Can you work these out from the model? Positions are in its coordinate system, mm. A direction names the side the tool comes from. Give positions to 0.01 mm unless a question says otherwise; leave off trailing zeros. Order: outer loops, then holes, each group sorted by start corner. A loop starts at its lowest first (then second) coordinate and runs counter-clockwise, first axis right, second up. Notation, with made-up numbers: M 5,58 L 13,58 A12 ccw 13,62 Z; hole C 64.5,42 d4. An arc over 180 degrees is marked long. Use a Markdown table: item, result. Add a question column.
from build123d import *

# Parameters (mm, degrees)
EXTRUDE1_DEPTH              = 12.7
ARC_MOUNTING_SLOT_I_DEPTH   = 56.885195213
CLAMPING_SCREW_HOLES_D      = 5.1054
CLAMPING_SCREW_HOLES_DEPTH  = 21.59
CLAMPING_SCREW_HOLES_TIP    = 1.533816902
SKETCH7_R                   = 9.525
CUT_EXTRUDE1_DEPTH          = 38.862
CUT_EXTRUDE2_DEPTH          = 25.4
ADVANCEDHOLE1_START         = -12.7
ADVANCEDHOLE1_OUTLINE_R     = 2.5527
ADVANCEDHOLE1_DEPTH         = 25.4
ADVANCEDHOLE1_2_OUTLINE_R   = 3.2639
ADVANCEDHOLE1_2_OUTLINE_R_2 = 2.5527
ADVANCEDHOLE1_2_DEPTH       = 11.1125
FILLET1_R                   = 1.5875


# Read off the part's stored shape, not the designer's step: AdvancedHole1
with BuildPart() as part:
    # Sketch1 → Extrude1 (new, symmetric)
    with BuildSketch(Plane.XY):
        Polygon((-28.575, 0), (-28.575, 6.35), (-38.1, 6.35), (-38.1, 16.1036), (-38.1, 54.9656), (-12.7, 54.9656), (10.16, 54.9656), (10.16, 33.3756), (0, 33.3756), (0, 16.1036), (12.7, 16.1036), (31.75, 16.1036), (31.75, 0), align=None)
    extrude(amount=EXTRUDE1_DEPTH, both=True)

    # Sketch2 → Arc mounting slot I (cut, through all)
    with BuildSketch(Plane(origin=(0, 16.1036, 0), x_dir=(-1, 0, 0), z_dir=(0, 1, 0))):
        with BuildLine():
            ThreePointArc((-25.839582785, -4.556215615), (-21.92608696, -7.296474893), (-19.185827683, -3.382979068))
            ThreePointArc((-19.185827683, -3.382979068), (-19.4818, 0), (-19.185827683, 3.382979068))
            ThreePointArc((-19.185827683, 3.382979068), (-21.92608696, 7.296474893), (-25.839582785, 4.556215615))
            ThreePointArc((-25.839582785, 4.556215615), (-26.2382, 0), (-25.839582785, -4.556215615))
        make_face()
    arc_mounting_slot_i = extrude(amount=-ARC_MOUNTING_SLOT_I_DEPTH, mode=Mode.SUBTRACT)

    # Arc mounting slot II: Arc mounting slot I across plane
    add(arc_mounting_slot_i.mirror(Plane(origin=(0, 0, 0), x_dir=(0, 0, 1), z_dir=(1, 0, 0))), mode=Mode.SUBTRACT)

    # Clamping screw holes
    with Locations(Plane(origin=(0, 54.9656, 0), x_dir=(-1, 0, 0), z_dir=(0, 1, 0))):
        with Locations((-3.96875, -7.9375), (-3.96875, 7.9375)):
            Hole(CLAMPING_SCREW_HOLES_D / 2, depth=CLAMPING_SCREW_HOLES_DEPTH)
            with Locations((0, 0, -(CLAMPING_SCREW_HOLES_DEPTH + CLAMPING_SCREW_HOLES_TIP / 2))):  # 118° drill point
                Cone(0, CLAMPING_SCREW_HOLES_D / 2, CLAMPING_SCREW_HOLES_TIP, mode=Mode.SUBTRACT)

    # Sketch7 → Cut-Extrude1 (cut)
    with BuildSketch(Plane(origin=(0, 54.9656, 0), x_dir=(1, 0, 0), z_dir=(0, 1, 0))):
        with Locations(Location((-19.05, 0, 0), (0, 0, 270))):
            Circle(SKETCH7_R)
    extrude(amount=-CUT_EXTRUDE1_DEPTH, mode=Mode.SUBTRACT)

    # Sketch9 → Cut-Extrude2 (cut)
    with BuildSketch(Plane.ZY.offset(38.1)):
        Polygon((-1.5875, 19.2786), (-1.5875, 54.9656), (1.5875, 54.9656), (1.5875, 16.1036), (-12.7, 16.1036), (-12.7, 19.2786), align=None)
    extrude(amount=-CUT_EXTRUDE2_DEPTH, mode=Mode.SUBTRACT)

    # AdvancedHole1 outline → AdvancedHole1 (cut)
    with BuildSketch(Plane.XY.offset(ADVANCEDHOLE1_START)):
        with Locations((-33.270888328, 37.1221)):
            Circle(ADVANCEDHOLE1_OUTLINE_R)
    extrude(amount=ADVANCEDHOLE1_DEPTH, mode=Mode.SUBTRACT)

    # AdvancedHole1 2 outline → AdvancedHole1 2 (cut)
    with BuildSketch(Plane.XY.offset(ADVANCEDHOLE1_START)):
        with Locations((-33.270888328, 37.1221)):
            Circle(ADVANCEDHOLE1_2_OUTLINE_R)
        with Locations((-33.270888328, 37.1221)):
            Circle(ADVANCEDHOLE1_2_OUTLINE_R_2, mode=Mode.SUBTRACT)
    extrude(amount=ADVANCEDHOLE1_2_DEPTH, mode=Mode.SUBTRACT)

    # Fillet1
    fillet1_edges = [part.edges().sort_by_distance(p)[0] for p in [
        (-12.7, 19.2786, -9.899757914),
        (-12.7, 16.1036, -9.899757914),
        (-33.270888328, 16.1036, 1.5875),
    ]]
    fillet(fillet1_edges, radius=FILLET1_R - 0.0001)  # a hair under: the kernel refuses the full size


solid = part.part
1. If we section it at D-D, the plane y = 14.5: List the corners of the cut face in (x, z) for me, then the cut area to 3 significant figures.
2. We'd pull the mould along Z, two halves only. Please class faces 6 (the face through (-19.48, 8.16, -0.05)), 7 (the face through (-10, 28, -12.7)), 8 (the face through (10.16, 44, 0)): +Z half, -Z half, draft (parallel to the pull), parting line (faces both ways), or undercut.
3. If we section it at B-B, the plane x = -23: List the corners of the cut face in (y, z) for me.
4. If we section it at A-A, the plane y = 5: List the corners of the cut face in (x, z) for me (3 decimals).
5. I need wall thicknesses on L1, parallel to X at y = 38.5, z = -4.5; L2, parallel to X at y = 38.5, z = -2; L3, parallel to Y at x = -33.5, z = 7. Which ranges of each line are inside material? Lowest first, please. Write a range as [from, to].
6. Will this pin go through, and if not, where does the flat tip stop? pin 1 (5 mm diameter, centred on x = -33, z = -5, fed in from -Y).
7. If we section it at C-C, the plane x = -16: List the corners of the cut face in (y, z) for me, then the cut area to 3 significant figures.
8. On a 3-axis mill with a long thin cutter (end or side, diameter ignored), from which of +Z, -Z, +X, -X, +Y, -Y can I reach the whole of each face in a straight line? I mean faces 1 (the face through (22, 8.16, -7.31)), 2 (the face through (-37, 37, 1.588)), 3 (the face through (-28.575, 3, 0)), 4 (the face through (-33.203, 16.556, 1.11)), 5 (the face through (-29, 19.279, -8)). Say none if no direction works.
Geometry results:
| question | item | result |
|---|---|---|
| 1 | outline | M -38.1,-12.7 L 31.75,-12.7 L 31.75,12.7 L -38.1,12.7 Z; hole M -25.84,-4.56 A3.38 ccw -19.19,-3.38 A19.48 cw -19.19,3.38 A3.38 ccw -25.84,4.56 A26.24 ccw Z; hole M 19.19,-3.38 A3.38 ccw 25.84,-4.56 A26.24 ccw 25.84,4.56 A3.38 ccw 19.19,3.38 A19.48 cw Z |
| 1 | area | 1,590 mm^2 |
| 2 | face 6 | undercut |
| 2 | face 7 | -Z half |
| 2 | face 8 | draft |
| 3 | outline | M 0,-12.7 L 16.1,-12.7 L 16.1,-7.31 L 0,-7.31 Z; M 0,7.31 L 16.1,7.31 L 16.1,8.67 L 54.97,8.67 L 54.97,12.7 L 0,12.7 Z; M 19.28,-12.7 L 54.97,-12.7 L 54.97,-8.67 L 19.28,-8.67 Z |
| 4 | outline | M -28.575,-12.7 L 31.75,-12.7 L 31.75,12.7 L -28.575,12.7 Z; hole M -25.84,-4.556 A3.378 ccw -19.186,-3.383 A19.482 cw -19.186,3.383 A3.378 ccw -25.84,4.556 A26.238 ccw Z; hole M 19.186,-3.383 A3.378 ccw 25.84,-4.556 A26.238 ccw 25.84,4.556 A3.378 ccw 19.186,3.383 A19.482 cw Z |
| 5 | L1 | x = [-38.1, -36.23], [-30.31, -27.44], [-10.66, 10.16] |
| 5 | L2 | x = [-38.1, -36.23], [-30.31, -28.36], [-9.74, 10.16] |
| 5 | L3 | y = [6.35, 34.58], [39.66, 54.97] |
| 6 | pin 1 | stops at y = 6.35 |
| 7 | outline | M 0,-12.7 L 16.1,-12.7 L 16.1,9.02 L 54.97,9.02 L 54.97,12.7 L 0,12.7 Z; M 19.28,-12.7 L 54.97,-12.7 L 54.97,-9.02 L 19.28,-9.02 Z |
| 7 | area | 683 mm^2 |
| 8 | face 1 | +Y, -Y |
| 8 | face 2 | -X, +Y |
| 8 | face 3 | +Z, -Z, -X, -Y |
| 8 | face 4 | -Z, -X, +Y |
| 8 | face 5 | -Z, -X |
